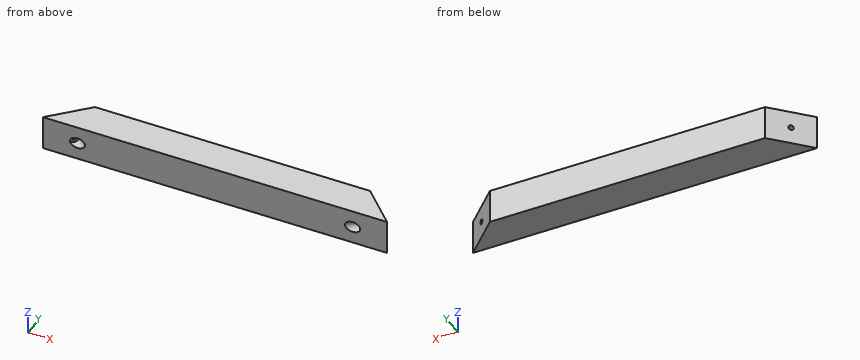
```python
from build123d import *

# Parameters (mm, degrees)
F1_DEPTH       = 80
F5_D           = 12
F5_CBORE_D     = 25
F5_CBORE_DEPTH = 40
F9_D           = 12
F9_CBORE_D     = 25
F9_CBORE_DEPTH = 40


with BuildPart() as f1:
    # F0 (on Top) → F1 (new body)
    with BuildSketch(Plane.XY):
        Polygon((320, 40), (-320, 40), (-400, -40), (400, -40), align=None)
    extrude(amount=F1_DEPTH)

    # F5 (through all)
    with Locations(Plane(origin=(-126.966991411, 126.966991411, 0), x_dir=(-0.7071067812, -0.7071067812, 0), z_dir=(0.7071067812, -0.7071067812, 0))):
        with Locations((254.5584412272, -40)):
            CounterBoreHole(F5_D / 2, F5_CBORE_D / 2, F5_CBORE_DEPTH)

    # F9 (through all)
    with Locations(Plane(origin=(126.966991411, 126.966991411, 0), x_dir=(-0.7071067812, 0.7071067812, 0), z_dir=(-0.7071067812, -0.7071067812, 0))):
        with Locations((-254.5584412272, -40)):
            CounterBoreHole(F9_D / 2, F9_CBORE_D / 2, F9_CBORE_DEPTH)


solid = f1.part
```
CAD build for the part. Positions are in the model's coordinates, mm. Give positions to 0.01 mm unless a question says otherwise; leave off trailing zeros. Loops run counter-clockwise (first coordinate to the right, second up) from the corner with the lowest first, then second, coordinate; pieces in that order, holes last. Notation, with made-up numbers: (56, -31.75) -> (70, -31.75) arc R22 cw to (70, -0.75) -> close; hole circle Ø2 at (9, 79.5). An arc over 180 degrees is marked (long way). Use a Markdown table: item, result.
1. Flat gauge pins, fed straight in: pin 1 (6 mm diameter, centred on y = 22, z = 65, fed in from +X); pin 2 (10 mm diameter, centred on y = 20, z = 9, fed in from +X); pin 3 (3 mm diameter, centred on y = 29.5, z = 58, fed in from +X). Where does each tip first touch, or does it go through?
Check result:
| item | result |
|---|---|
| pin 1 | stops at x = 341 |
| pin 2 | stops at x = 345 |
| pin 3 | stops at x = 332 |
2. Slice it at A-A (z = 68). List the corners of the cut face in (x, y), plus the area to 3 significant figures.
Check result:
| item | result |
|---|---|
| outline | (-400, -40) -> (400, -40) -> (320, 40) -> (-320, 40) -> close |
| area | 57,600 mm^2 |
3. Slice it at B-B (y = 29). List the corners of the cut face in (x, z), plus the area to 3 significant figures.
Check result:
| item | result |
|---|---|
| outline | (-331, 0) -> (331, 0) -> (331, 80) -> (-331, 80) -> close |
| area | 53,000 mm^2 |
4. Wall check: L1, parallel to Z at x = -323.5, y = -22.5; L2, parallel to Z at x = 317, y = -35.5; L3, parallel to X at y = 17.5, z = 16.5. Give the ranges that are in metal, low to high. Write a range as [from, to].
Check result:
| item | result |
|---|---|
| L1 | z = [0, 32.37], [47.63, 80] |
| L2 | z = [0, 28.68], [51.32, 80] |
| L3 | x = [-342.5, 342.5] |
